For this review, use the dimensioned drawing (mm, ordinates from the lowest corner) and the shaded views. Round coordinates to 2 decimals unless told otherwise and drop trailing zeros. Loops run counter-clockwise (first coordinate to the right, second up) from the corner with the lowest first, then second, coordinate; pieces in that order, holes last. Notation, with made-up numbers: (32, -40) -> (52, -40) arc R27 cw to (52, -16) -> close; hole circle Ø5 at (-5.75, 0.5). An arc over 180 degrees is marked (long way). Answer as CSV lines item,"result". Start each with the question number.
(1) Take a section at C-C, the plane x = 45. Write out the cut boundary in (y, z), and give its area (4 significant figures).
(2) To check wall thickness, follow line 1 (Y direction, x = 57.5, z = 2.35); line 2 (Y direction, x = 24, z = 2.5); line 3 (X direction, y = 41.5, z = 2). State the ranges of each line that lie inside material, in increasing order. Write a range as from..to.
(3) Take a section at A-A, the plane x = 7.5. Write out the cut boundary in (y, z).
(4) Take a section at D-D, the plane y = 38. Write out the cut boundary in (x, z), and give its area (4 significant figures).
(5) Take a section at B-B, the plane y = 77.5. Write out the cut boundary in (x, z).
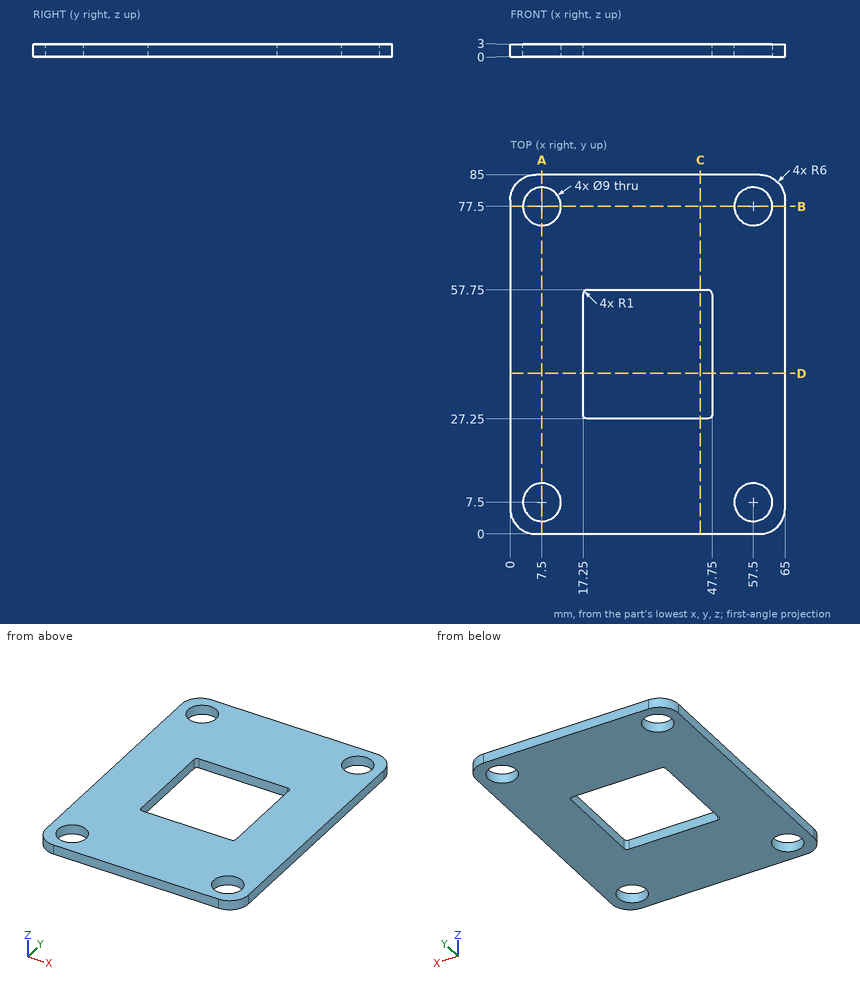
The answers:
1,outline,"(0, 0) -> (27.25, 0) -> (27.25, 3) -> (0, 3) -> close; (57.75, 0) -> (85, 0) -> (85, 3) -> (57.75, 3) -> close"
1,area,"163.5 mm²"
2,line 1,"0..3, 12..73, 82..85"
2,line 2,"0..27.25, 57.75..85"
2,line 3,"0..17.25, 47.75..65"
3,outline,"(0, 0) -> (3, 0) -> (3, 3) -> (0, 3) -> close; (12, 0) -> (73, 0) -> (73, 3) -> (12, 3) -> close; (82, 0) -> (85, 0) -> (85, 3) -> (82, 3) -> close"
4,outline,"(0, 0) -> (17.25, 0) -> (17.25, 3) -> (0, 3) -> close; (47.75, 0) -> (65, 0) -> (65, 3) -> (47.75, 3) -> close"
4,area,"103.5 mm²"
5,outline,"(0, 0) -> (3, 0) -> (3, 3) -> (0, 3) -> close; (12, 0) -> (53, 0) -> (53, 3) -> (12, 3) -> close; (62, 0) -> (65, 0) -> (65, 3) -> (62, 3) -> close"
